```python
from build123d import *

# Parameters (mm, degrees)
TRACK_START     = -3.75
TRACK_OUTLINE_R = 85
TRACK_DEPTH     = 7.5
SKETCH2_R       = 87
SKETCH2_R_2     = 83
RAIL_DEPTH      = 1


# Read off the part's stored shape, not the designer's step: Track
with BuildPart() as part:
    # Track outline → Track (new body)
    with BuildSketch(Plane.XY.offset(TRACK_START)):
        Circle(TRACK_OUTLINE_R)
        with BuildLine():
            Line((57.25, -60.095236916), (57.25, -13.13))
            Line((57.25, -13.13), (49.25, -13.13))
            Line((49.25, -13.13), (49.25, -66.808962722))
            ThreePointArc((49.25, -66.808962722), (-63.578054165, -53.355702868), (-57.25, 60.095236916))
            Line((-57.25, 60.095236916), (-57.25, 13.13))
            Line((-57.25, 13.13), (-49.25, 13.13))
            Line((-49.25, 13.13), (-49.25, 66.808962722))
            ThreePointArc((-49.25, 66.808962722), (63.578054165, 53.355702868), (57.25, -60.095236916))
        make_face(mode=Mode.SUBTRACT)
    extrude(amount=TRACK_DEPTH)

    # Sketch2 → Rail (add)
    with BuildSketch(Plane.XY.offset(3.75)):
        Circle(SKETCH2_R)
        with Locations(Location((0, 0, 0), (0, 0, 133.611037517))):
            Circle(SKETCH2_R_2, mode=Mode.SUBTRACT)
    rail = extrude(amount=RAIL_DEPTH)

    # Mirror1: Rail across plane
    add(rail.mirror(Plane.XY))


solid = part.part
```
Read the model definition and answer for the solid it produces. Units are mm, in the model's axes. A direction names the side the tool comes from. Round coordinates to 2 decimals unless told otherwise and drop trailing zeros. Write each loop counter-clockwise with the first axis right and the second up, starting at its lowest first coordinate (ties: lowest second). Pieces come first, ordered by that corner, then holes. Notation, with made-up numbers: M 37.5,48 L 45.5,48 A13 cw 45.5,70 Z; hole C 12,-20.75 d2. An arc over 180 degrees is marked long. One line per item, written item: value.
Q1. Find section D-D on y = 26.5. Write down the section's boundary in (x, z).
Data:
outline: M -82.87,-4.75 L -78.66,-4.75 L -78.66,4.75 L -82.87,4.75 L -82.87,3.75 L -80.76,3.75 L -80.76,-3.75 L -82.87,-3.75 Z; M -57.25,-3.75 L -49.25,-3.75 L -49.25,3.75 L -57.25,3.75 Z; M 78.66,-4.75 L 82.87,-4.75 L 82.87,-3.75 L 80.76,-3.75 L 80.76,3.75 L 82.87,3.75 L 82.87,4.75 L 78.66,4.75 Z
Q2. Straight lines are drawn through the part: line 1 (Y direction, x = 0, z = -4.1); line 2 (X direction, y = -38, z = 3.5); line 3 (X direction, y = -39, z = -2.5). For each, find the intervals that lie inside material, in ascending order. Write a range as [from, to].
Data:
line 1: [-87, -83], [83, 87]
line 2: [-76.03, -73.79], [49.25, 57.25], [73.79, 76.03]
line 3: [-75.52, -73.27], [49.25, 57.25], [73.27, 75.52]
Q3. Find section A-A on y = 0. Write down the section's boundary in (x, z).
Data:
outline: M -87,-4.75 L -83,-4.75 L -83,4.75 L -87,4.75 L -87,3.75 L -85,3.75 L -85,-3.75 L -87,-3.75 Z; M 83,-4.75 L 87,-4.75 L 87,-3.75 L 85,-3.75 L 85,3.75 L 87,3.75 L 87,4.75 L 83,4.75 Z
Q4. For a pull along Y with two mould halves and no side action, classify faces 6 (the cylindrical face through (-67.453, -51.721, -0.053)), 7 (the flat face through (77, -32, -4.75)), 8 (the flat face through (53, -13.13, 0)) as +Y half, -Y half, draft (parallel to the pull), parting line (faces both ways), or undercut.
Data:
face 6: parting line
face 7: draft
face 8: undercut
Q5. Which of the six approach directions +Z, -Z, +X, -X, +Y, -Y give full straight-line access (tool end or side, diameter ignored) to faces 1 (the flat face through (53, -40, 3.75)), 2 (the flat face through (18.9, -83.4, 3.75)), 3 (the flat face through (77, -32, 4.75)), 4 (the flat face through (-53, 40, -3.75)), 5 (the flat face through (-57.25, 37, 0))?
Data:
face 1: +Z
face 2: none
face 3: +Z, +X, -X, +Y, -Y
face 4: -Z
face 5: +Z, -Z
Q6. Flat-ended cylindrical pins translate along their axes: pin 1 Ø2 at (y, z) = (-13, 1) entering from +X; pin 2 Ø3 at (x, z) = (60.5, -1) entering from +Y; pin 3 Ø6.5 at (x, y) = (55, -50.5) entering from +Z; pin 4 Ø3 at (x, y) = (49, -11.5) entering from +Z. Find the tip coordinate at first contact, or state that the pin passes through.
Data:
pin 1: x = 84.15
pin 2: y = 61.19
pin 3: z = 3.75
pin 4: through
Q7. Find section C-C on z = -2.25. Write down the section's boundary in (x, y).
Data:
outline: C 0,0 d170; hole M -57.25,13.13 L -57.25,60.1 A83 ccw 49.25,-66.81 L 49.25,-13.13 L 57.25,-13.13 L 57.25,-60.1 A83 ccw -49.25,66.81 L -49.25,13.13 Z
